Build history of the part. All positions in model axes, mm. A direction names the side the tool comes from. Round coordinates to 2 decimals unless told otherwise and drop trailing zeros. Write each loop counter-clockwise with the first axis right and the second up, starting at its lowest first coordinate (ties: lowest second). Pieces come first, ordered by that corner, then holes. Notation, with made-up numbers: M -5.5,89.25 L 39.5,89.25 A24 ccw 39.5,111.25 Z; hole C 3,4 d5. An arc over 180 degrees is marked long. Use a Markdown table: item, result.
from build123d import *

# Parameters (mm, degrees)
EXTRUDE_1_DEPTH = 200
FILLET_1_R      = 22.5
FILLET_2_R      = 7.5


with BuildPart() as part:
    # ｽｹｯﾁ5 → ﾎﾞｽ - 押し出し1 (new body)
    with BuildSketch(Plane(origin=(0, 0, 0), x_dir=(1, 0, 0), z_dir=(0, 1, 0))):
        Polygon((0, 0), (120, 0), (120, 30), (105, 30), (105, 15), (67.5, 15), (67.5, 105), (105, 105), (105, 90), (120, 90), (120, 120), (0, 120), (0, 90), (15, 90), (15, 105), (52.5, 105), (52.5, 15), (15, 15), (15, 30), (0, 30), align=None)
    extrude(amount=EXTRUDE_1_DEPTH)

    # ﾌｨﾚｯﾄ1
    fillet_1_edges = [part.edges().sort_by_distance(p)[0] for p in [
        (0, 100, -120),
        (120, 100, -120),
        (120, 100, 0),
        (0, 100, 0),
    ]]
    fillet(fillet_1_edges, radius=FILLET_1_R)

    # ﾌｨﾚｯﾄ2
    fillet_2_edges = [part.edges().sort_by_distance(p)[0] for p in [
        (15, 100, -15),
        (15, 100, -105),
        (105, 100, -105),
        (105, 100, -15),
    ]]
    fillet(fillet_2_edges, radius=FILLET_2_R)


solid = part.part
Q1. Cut at D-D on x = 101. Give the cut face in (y, z), and give its area (3 significant figures).
Response values:
| item | result |
|---|---|
| outline | M 0,-119.73 L 200,-119.73 L 200,-104.13 L 0,-104.13 Z; M 0,-15.87 L 200,-15.87 L 200,-0.27 L 0,-0.27 Z |
| area | 6,240 mm2 |
Q2. Drop flat-ended pins along their axis: P1, Ø4.5, axis at x = 6.5, y = 105.5, coming from the -Z side; P2, Ø1.5, axis at y = 42.5, z = -84.5, coming from the -X side; P3, Ø12, axis at x = 14, y = 143, coming from the +Z side; P4, Ø4, axis at x = 14, z = -94, coming from the -Y side. Give the stop position or say it passes through.
Response values:
| item | result |
|---|---|
| P1 | stops at z = -115.31 |
| P2 | stops at x = 52.5 |
| P3 | stops at z = -0.14 |
| P4 | stops at y = 0 |
Q3. Cut at C-C on y = 90. Give the cut face in (x, z), and give its area (3 significant figures).
Response values:
| item | result |
|---|---|
| outline | M 0,-97.5 A22.5 ccw 22.5,-120 L 97.5,-120 A22.5 ccw 120,-97.5 L 120,-90 L 105,-90 L 105,-97.5 A7.5 cw 97.5,-105 L 67.5,-105 L 67.5,-15 L 97.5,-15 A7.5 cw 105,-22.5 L 105,-30 L 120,-30 L 120,-22.5 A22.5 ccw 97.5,0 L 22.5,0 A22.5 ccw 0,-22.5 L 0,-30 L 15,-30 L 15,-22.5 A7.5 cw 22.5,-15 L 52.5,-15 L 52.5,-105 L 22.5,-105 A7.5 cw 15,-97.5 L 15,-90 L 0,-90 Z |
| area | 5,460 mm2 |
Q4. Cut at B-B on x = 17.5. Give the cut face in (y, z), and give its area (3 significant figures).
Response values:
| item | result |
|---|---|
| outline | M 0,-119.44 L 200,-119.44 L 200,-103.09 L 0,-103.09 Z; M 0,-16.91 L 200,-16.91 L 200,-0.56 L 0,-0.56 Z |
| area | 6,540 mm2 |
Q5. Two-plate mould, pull along X, no slides. Class faces 1 (the flat face through (82, 99, -105)), 2 (the flat face through (0, 99, -26)), 3 (the flat face through (113, 99, -30)): +X half, -X half, draft (parallel to the pull), parting line (faces both ways), or undercut.
Response values:
| item | result |
|---|---|
| face 1 | undercut |
| face 2 | -X half |
| face 3 | draft |
Q6. Cut at A-A on z = -94.5. Give the cut face in (x, y), and give its area (3 significant figures).
Response values:
| item | result |
|---|---|
| outline | M 0,0 L 15,0 L 15,200 L 0,200 Z; M 52.5,0 L 67.5,0 L 67.5,200 L 52.5,200 Z; M 105,0 L 120,0 L 120,200 L 105,200 Z |
| area | 9,000 mm2 |
Q7. Drill centre lines: L1, parallel to X at y = 96, z = -93; L2, parallel to Z at x = 50, y = 187; L3, parallel to X at y = 32.5, z = -101.5. Where is each one in solid material? Low to high.
Response values:
| item | result |
|---|---|
| L1 | x = 0 to 15, 52.5 to 67.5, 105 to 120 |
| L2 | z = -120 to -105, -15 to 0 |
| L3 | x = 0.36 to 16.16, 52.5 to 67.5, 103.84 to 119.64 |
Q8. Which spindle directions (+Z, -Z, +X, -X, +Y, -Y) get a long thin tool onto all of the face, cutting with end or side? Do faces 4 (the flat face through (52.5, 99, -61)), 5 (the flat face through (8, 99, -30)), 6 (the flat face through (60, 0, -60)). Say none if no direction does.
Response values:
| item | result |
|---|---|
| face 4 | +Y, -Y |
| face 5 | -X, +Y, -Y |
| face 6 | +Z, -Z, +X, -X, -Y |
